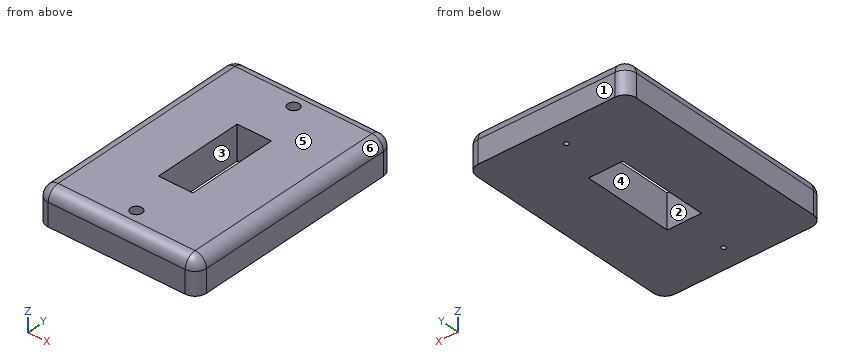
```python
from build123d import *

# Parameters (mm, degrees)
SKETCH1_W           = 70
SKETCH1_H           = 100
BOSS_EXTRUDE1_DEPTH = 15
SKETCH3_W           = 15
SKETCH3_H           = 40
CUT_EXTRUDE1_DEPTH  = 63.84902545
SKETCH4_R           = 2.5
CUT_EXTRUDE2_DEPTH  = 63.84902545
FILLET1_R           = 5
BOSS_EXTRUDE2_START = -2
SKETCH5_R           = 2.5
SKETCH5_R_2         = 1
BOSS_EXTRUDE2_DEPTH = 2
FILLET2_R           = 5


with BuildPart() as part:
    # Sketch1 → Boss-Extrude1 (new body)
    with BuildSketch(Plane.XY):
        Rectangle(SKETCH1_W, SKETCH1_H)
    extrude(amount=BOSS_EXTRUDE1_DEPTH)

    # Sketch3 → Cut-Extrude1 (cut, through all)
    with BuildSketch(Plane.XY.offset(15)):
        Rectangle(SKETCH3_W, SKETCH3_H)
    extrude(amount=-CUT_EXTRUDE1_DEPTH, mode=Mode.SUBTRACT)

    # Sketch4 → Cut-Extrude2 (cut, through all)
    with BuildSketch(Plane.XY.offset(15)):
        with Locations((0, -40)):
            Circle(SKETCH4_R)
        with Locations((0, 40)):
            Circle(SKETCH4_R)
    extrude(amount=-CUT_EXTRUDE2_DEPTH, mode=Mode.SUBTRACT)

    # Fillet1
    fillet1_edges = [part.edges().sort_by_distance(p)[0] for p in [
        (-35, 0, 15),
        (0, -50, 15),
        (35, 0, 15),
        (0, 50, 15),
    ]]
    fillet(fillet1_edges, radius=FILLET1_R)

    # Sketch5 → Boss-Extrude2 (add)
    # profile 1 of 2: a face of its own
    with BuildSketch(Plane(origin=(0, 0, 0), x_dir=(-1, 0, 0), z_dir=(0, 0, -1)).offset(BOSS_EXTRUDE2_START)):
        with Locations(Location((0, 40, 0), (0, 0, 180))):
            Circle(SKETCH5_R)
        with Locations((0, 40)):
            Circle(SKETCH5_R_2, mode=Mode.SUBTRACT)
    # profile 2 of 2: a face of its own
    with BuildSketch(Plane(origin=(0, 0, 0), x_dir=(-1, 0, 0), z_dir=(0, 0, -1)).offset(BOSS_EXTRUDE2_START)):
        with Locations(Location((0, -40, 0), (0, 0, 180))):
            Circle(SKETCH5_R)
        with Locations((0, -40)):
            Circle(SKETCH5_R_2, mode=Mode.SUBTRACT)
    extrude(amount=BOSS_EXTRUDE2_DEPTH)

    # Fillet2
    # the kernel refuses this fillet: 5 mm, written as the material it takes off along each edge
    with BuildSketch(Plane(origin=(-30, 45, 10), x_dir=(0, 1, 0), z_dir=(-1, 0, 0))) as fillet2_piece_1_section:
        Polygon((0, 0), (FILLET2_R, 0), (FILLET2_R, -FILLET2_R), (0, -FILLET2_R), align=None)
    fillet2_piece_1 = extrude(amount=FILLET2_R, mode=Mode.PRIVATE)
    fillet2_piece_1 = fillet2_piece_1 - Plane(origin=(-30, 45, 10), x_dir=(0, -0.7071067811865475, -0.7071067811865475), z_dir=(-1, 0, 0)) * Sphere(FILLET2_R, mode=Mode.PRIVATE)
    add(fillet2_piece_1, mode=Mode.SUBTRACT)
    with BuildSketch(Plane(origin=(30, 45, 10), x_dir=(0, 1, 0), z_dir=(1, 0, 0))) as fillet2_piece_2_section:
        Polygon((0, 0), (FILLET2_R, 0), (FILLET2_R, FILLET2_R), (0, FILLET2_R), align=None)
    fillet2_piece_2 = extrude(amount=FILLET2_R, mode=Mode.PRIVATE)
    fillet2_piece_2 = fillet2_piece_2 - Plane(origin=(30, 45, 10), x_dir=(0, -0.7071067811865475, -0.7071067811865475), z_dir=(1, 0, 0)) * Sphere(FILLET2_R, mode=Mode.PRIVATE)
    add(fillet2_piece_2, mode=Mode.SUBTRACT)
    with BuildSketch(Plane(origin=(-30, -45, 10), x_dir=(-1, 0, 0), z_dir=(0, -1, 0))) as fillet2_piece_3_section:
        Polygon((0, 0), (FILLET2_R, 0), (FILLET2_R, -FILLET2_R), (0, -FILLET2_R), align=None)
    fillet2_piece_3 = extrude(amount=FILLET2_R, mode=Mode.PRIVATE)
    fillet2_piece_3 = fillet2_piece_3 - Plane(origin=(-30, -45, 10), x_dir=(0.7071067811865475, 0, -0.7071067811865475), z_dir=(0, -1, 0)) * Sphere(FILLET2_R, mode=Mode.PRIVATE)
    add(fillet2_piece_3, mode=Mode.SUBTRACT)
    with BuildSketch(Plane(origin=(30, -45, 10), x_dir=(1, 0, 0), z_dir=(0, -1, 0))) as fillet2_piece_4_section:
        Polygon((0, 0), (FILLET2_R, 0), (FILLET2_R, FILLET2_R), (0, FILLET2_R), align=None)
    fillet2_piece_4 = extrude(amount=FILLET2_R, mode=Mode.PRIVATE)
    fillet2_piece_4 = fillet2_piece_4 - Plane(origin=(30, -45, 10), x_dir=(-0.7071067811865475, 0, -0.7071067811865475), z_dir=(0, -1, 0)) * Sphere(FILLET2_R, mode=Mode.PRIVATE)
    add(fillet2_piece_4, mode=Mode.SUBTRACT)
    with BuildSketch(Plane(origin=(35, -50, -12.5), x_dir=(-1, 0, 0), z_dir=(0, 0, 1)), Plane(origin=(35, 50, -12.5), x_dir=(0, -1, 0), z_dir=(0, 0, 1))) as fillet2_piece_5:
        with BuildLine():
            CenterArc((FILLET2_R, -FILLET2_R), FILLET2_R, 90, 90)
            Line((0, -FILLET2_R), (0, 0))
            Line((0, 0), (FILLET2_R, 0))
        make_face()
    extrude(amount=22.5, mode=Mode.SUBTRACT)
    with BuildSketch(Plane(origin=(-35, -50, -12.5), x_dir=(1, 0, 0), z_dir=(0, 0, 1)), Plane(origin=(-35, 50, -12.5), x_dir=(0, -1, 0), z_dir=(0, 0, 1))) as fillet2_piece_6:
        with BuildLine():
            CenterArc((FILLET2_R, FILLET2_R), FILLET2_R, 180, 90)
            Line((0, FILLET2_R), (0, 0))
            Line((0, 0), (FILLET2_R, 0))
        make_face()
    extrude(amount=22.5, mode=Mode.SUBTRACT)


solid = part.part
```
Geometry: final body of the model. Coordinates: model frame, mm. Face numbers are marked on the shaded views. A direction names the side the tool comes from. Coordinates: 2 decimals unless noted, no trailing zeros. Order: outer loops, then holes, each group sorted by start corner. A loop starts at its lowest first (then second) coordinate and runs counter-clockwise, first axis right, second up. Notation, with made-up numbers: (47, 38.25) - (81, 38.25) arc R36 cw to (81, 74.25) - close; hole circle Ø11 at (85, 15.25). An arc over 180 degrees is marked (long way). Write each question's results on one line, items separated by ' | '.
(1) Mould query, pull axis X, two halves, no side actions, for the marked faces 3, 4, 5 and 6. Classes: +X half, -X half, draft (parallel to the pull), parting line (faces both ways), or undercut.
Values found:
face 3: undercut | face 4: undercut | face 5: draft | face 6: +X half
(2) Section query A-A, the plane y = 40. Return the cut outline in (x, z), plus the area to 3 significant figures.
Values found:
outline: (-35, 0) - (-1, 0) - (-1, 2) - (-2.5, 2) - (-2.5, 15) - (-30, 15) arc R5 ccw to (-35, 10) - close; (1, 0) - (35, 0) - (35, 10) arc R5 ccw to (30, 15) - (2.5, 15) - (2.5, 2) - (1, 2) - close | area: 970 mm²
(3) Set-up query: the marked faces 1 and 2. Return all of +Z, -Z, +X, -X, +Y, -Y with unobstructed straight access to the full face (end or side cutting, diameter ignored); none if empty.
Values found:
face 1: +Z, -Z, +X, -X, +Y | face 2: +Z, -Z
(4) Line query: line 1 (Y direction, x = 0, z = 1); line 2 (Y direction, x = 0, z = 10); line 3 (X direction, y = -15, z = 8.5). Output: solid intervals per line, ascending. Write a range as [from, to].
Values found:
line 1: y = [-50, -41], [-39, -20], [20, 39], [41, 50] | line 2: y = [-50, -42.5], [-37.5, -20], [20, 37.5], [42.5, 50] | line 3: x = [-35, -7.5], [7.5, 35]
(5) Section query C-C, the plane z = 12. Return the cut outline in (x, y).
Values found:
outline: (-34.58, -45) arc R4.58 ccw to (-30, -49.58) - (30, -49.58) arc R4.58 ccw to (34.58, -45) - (34.58, 45) arc R4.58 ccw to (30, 49.58) - (-30, 49.58) arc R4.58 ccw to (-34.58, 45) - close; hole (-7.5, -20) - (7.5, -20) - (7.5, 20) - (-7.5, 20) - close; hole circle Ø5 at (0, -40); hole circle Ø5 at (0, 40)
(6) First-contact query: pin 1 Ø6.5 at (x, y) = (0, -40) entering from +Z; pin 2 Ø3 at (x, y) = (0, -40) entering from +Z. Flat tips, straight axial feed; report the tip coordinate or a pass-through.
Values found:
pin 1: stops at z = 15 | pin 2: stops at z = 2
(7) Section query B-B, the plane x = 0. Return the cut outline in (y, z), plus the area to 3 significant figures.
Values found:
outline: (-50, 0) - (-41, 0) - (-41, 2) - (-42.5, 2) - (-42.5, 15) - (-45, 15) arc R5 ccw to (-50, 10) - close; (-39, 0) - (-20, 0) - (-20, 15) - (-37.5, 15) - (-37.5, 2) - (-39, 2) - close; (20, 0) - (39, 0) - (39, 2) - (37.5, 2) - (37.5, 15) - (20, 15) - close; (41, 0) - (50, 0) - (50, 10) arc R5 ccw to (45, 15) - (42.5, 15) - (42.5, 2) - (41, 2) - close | area: 751 mm²
